Could you check a few things on this model? Use its own coordinates, in mm. A direction names the side the tool comes from. Coordinates: 2 decimals unless noted, no trailing zeros. Loops run counter-clockwise (first coordinate to the right, second up) from the corner with the lowest first, then second, coordinate; pieces in that order, holes last. Notation, with made-up numbers: (-20.5, -9.75) -> (-8.5, -9.75) arc R22 cw to (-8.5, 28.25) -> close; hole circle Ø1 at (-34.5, 89). An arc over 180 degrees is marked (long way). One line per question, with ' | ' between items.
from build123d import *

# Parameters (mm, degrees)
SKETCH3_W                   = 65
SKETCH3_H                   = 100
BOSS_EXTRUDE1_DEPTH         = 40
F_21_0_159_DIAMETER_HOLE1_D = 4.0386
SHELL1_T                    = -3.5
FILLET1_R                   = 2
SKETCH14_W                  = 13
SKETCH14_H                  = 7
CUT_EXTRUDE1_DEPTH          = 10
FILLET2_R                   = 5
CHAMFER2_SIZE               = 4
SKETCH15_R                  = 6.4
CUT_EXTRUDE3_DEPTH          = 10
SKETCH17_R                  = 6.4
CUT_EXTRUDE6_DEPTH          = 10
CUT_EXTRUDE8_DEPTH          = 1.5
SKETCH20_W                  = 51
SKETCH20_H                  = 53
BOSS_EXTRUDE3_DEPTH         = 17
SKETCH22_W                  = 49
SKETCH22_H                  = 49
CUT_EXTRUDE9_DEPTH          = 17
SKETCH23_R                  = 2.5
CUT_EXTRUDE10_DEPTH         = 3


with BuildPart() as part:
    # Sketch3 → Boss-Extrude1 (new body)
    with BuildSketch(Plane(origin=(0, 0, 0), x_dir=(1, 0, 0), z_dir=(0, 1, 0))):
        Rectangle(SKETCH3_W, SKETCH3_H)
    extrude(amount=BOSS_EXTRUDE1_DEPTH)

    # #21 (0.159) Diameter Hole1 (through all)
    with Locations(Plane(origin=(0, 40, 0), x_dir=(1, 0, 0), z_dir=(0, 1, 0))):
        with Locations((-26.15, 43.65), (26.15, 43.65), (26.15, -43.65), (-26.15, -43.65)):
            Hole(F_21_0_159_DIAMETER_HOLE1_D / 2)

    # Shell1
    shell1_openings = [part.faces().sort_by_distance(p)[0] for p in [
        (0, 40, 0),
    ]]
    offset(amount=SHELL1_T, openings=shell1_openings, kind=Kind.INTERSECTION)

    # Fillet1
    fillet1_edges = [part.edges().sort_by_distance(p)[0] for p in [
        (29, 21.75, 38.923460834),
        (21.423460834, 21.75, -46.5),
        (-29, 21.75, -38.923460834),
        (-21.423460834, 21.75, 46.5),
        (-29, 21.75, 38.923460834),
        (21.423460834, 21.75, 46.5),
        (29, 21.75, -38.923460834),
        (-21.423460834, 21.75, -46.5),
    ]]
    fillet(fillet1_edges, radius=FILLET1_R)

    # Sketch14 → Cut-Extrude1 (cut)
    with BuildSketch(Plane(origin=(0, 0, 0), x_dir=(1, 0, 0), z_dir=(0, 1, 0))):
        with Locations((-8.88380044, -40.5)):
            Rectangle(SKETCH14_W, SKETCH14_H)
        with Locations((9.11619956, -40.5)):
            Rectangle(SKETCH14_W, SKETCH14_H)
        with Locations((-8.88380044, 26.688454416)):
            Rectangle(SKETCH14_W, SKETCH14_H)
        with Locations((9.11619956, 26.688454416)):
            Rectangle(SKETCH14_W, SKETCH14_H)
    extrude(amount=CUT_EXTRUDE1_DEPTH, mode=Mode.SUBTRACT)

    # Fillet2
    fillet2_edges = [part.edges().sort_by_distance(p)[0] for p in [
        (32.5, 20, 50),
        (-32.5, 20, 50),
        (-32.5, 20, -50),
        (32.5, 20, -50),
    ]]
    fillet(fillet2_edges, radius=FILLET2_R)

    # Chamfer2
    chamfer2_edges = [part.edges().sort_by_distance(p)[0] for p in [
        (-31.035533906, 0, -48.535533906),
        (-31.035533906, 0, 48.535533906),
        (31.035533906, 0, -48.535533906),
        (31.035533906, 0, 48.535533906),
        (32.5, 0, 0),
    ]]
    chamfer(chamfer2_edges, length=CHAMFER2_SIZE)

    # Sketch15 → Cut-Extrude3 (cut)
    with BuildSketch(Plane(origin=(0, 0, -50), x_dir=(-1, 0, 0), z_dir=(0, 0, -1))):
        with Locations((0, 22)):
            Circle(SKETCH15_R)
    extrude(amount=-CUT_EXTRUDE3_DEPTH, mode=Mode.SUBTRACT)

    # Sketch17 → Cut-Extrude6 (cut)
    with BuildSketch(Plane(origin=(32.5, 0, 0), x_dir=(0, 0, -1), z_dir=(1, 0, 0))):
        with Locations((26.233387705, 29.113582019)):
            Circle(SKETCH17_R)
    extrude(amount=-CUT_EXTRUDE6_DEPTH, mode=Mode.SUBTRACT)

    # Sketch18 → Cut-Extrude8 (cut)
    with BuildSketch(Plane(origin=(0, 3.5, 0), x_dir=(1, 0, 0), z_dir=(0, 1, 0))):
        with BuildLine():
            Line((2.962903006, 35.660547198), (3, 35.660547198))
            Line((3, 35.660547198), (3, 31.660547198))
            Line((3, 31.660547198), (-3, 31.660547198))
            Line((-3, 31.660547198), (-3, 35.660547198))
            Line((-3, 35.660547198), (-2.962903006, 35.660547198))
            ThreePointArc((-2.962903006, 35.660547198), (0, 46.338397214), (2.962903006, 35.660547198))
        make_face()
    extrude(amount=-CUT_EXTRUDE8_DEPTH, mode=Mode.SUBTRACT)

    # Sketch20 → Boss-Extrude3 (add)
    with BuildSketch(Plane(origin=(0, 3.5, 0), x_dir=(1, 0, 0), z_dir=(0, 1, 0))):
        with Locations((3.5, -6.305895328)):
            Rectangle(SKETCH20_W, SKETCH20_H)
    extrude(amount=BOSS_EXTRUDE3_DEPTH)

    # Sketch22 → Cut-Extrude9 (cut)
    with BuildSketch(Plane(origin=(0, 20.5, 0), x_dir=(1, 0, 0), z_dir=(0, 1, 0))):
        with Locations((4.5, -6.305895328)):
            Rectangle(SKETCH22_W, SKETCH22_H)
    extrude(amount=-CUT_EXTRUDE9_DEPTH, mode=Mode.SUBTRACT)

    # Sketch23 → Cut-Extrude10 (cut)
    with BuildSketch(Plane.XY.offset(-18.194104672)):
        with Locations((-16.3, 8.5)):
            Circle(SKETCH23_R)
        with Locations((0, 8.5)):
            Circle(SKETCH23_R)
        with Locations((16.3, 8.5)):
            Circle(SKETCH23_R)
    extrude(amount=-CUT_EXTRUDE10_DEPTH, mode=Mode.SUBTRACT)


solid = part.part
1) I'm going to push flat-ended pins straight in: pin 1 Ø1.8 at (x, y) = (8.5, 1.5) entering from -Z; pin 2 Ø5 at (x, z) = (-18, 15) entering from +Y; pin 3 Ø1.6 at (y, z) = (2.5, -34) entering from +X. Where does each tip first touch, or does it pass through?
Data:
pin 1: z = -48.4 | pin 2: y = 20.5 | pin 3: x = 31.8
2) On a 3-axis mill with a long thin cutter (end or side, diameter ignored), from which of +Z, -Z, +X, -X, +Y, -Y can I reach the whole of each face in a straight line? I mean faces 4 (the face through (9, 2, 37)), 5 (the face through (-22, 12, 7)), 6 (the face through (-0.54, 6.06, -19.18)). Say none if no direction works.
Data:
face 4: +Y, -Y | face 5: +Y | face 6: none
3) If we section it at A-A on x = 10.5: Please give me the cut outline in (y, z).
Data:
outline: (0, -46) -> (4, -50) -> (40, -50) -> (40, -46.5) -> (3.5, -46.5) -> (3.5, -30.19) -> (0, -30.19) -> close; (0, -23.19) -> (3.5, -23.19) -> (3.5, -20.19) -> (20.5, -20.19) -> (20.5, -18.19) -> (3.5, -18.19) -> (3.5, 30.81) -> (20.5, 30.81) -> (20.5, 32.81) -> (3.5, 32.81) -> (3.5, 37) -> (0, 37) -> close; (0, 44) -> (3.5, 44) -> (3.5, 46.5) -> (40, 46.5) -> (40, 50) -> (4, 50) -> (0, 46) -> close
4) We'd pull the mould along Z, two halves only. Please class faces 1 (the face through (-29.62, 1.97, -47.08)), 2 (the face through (-29.58, 1.97, 47.12)), 3 (the face through (20, 21, -46)): pulls with the +Z half, pulls with the -Z half, needs draft (parallel to the pull), parting line crosses it, or undercut.
Data:
face 1: pulls with the -Z half | face 2: pulls with the +Z half | face 3: undercut
5) If we section it at C-C on y = 8.5: Give the number of separate pieces and of enclosed holes in the cut face, and give its area (3 significant figures).
Data:
separate pieces: 3 | enclosed holes: 5 | area: 1,570 mm²
6) I need wall thicknesses on line 1 along X through (y, z) = (15, 13); line 2 along Z through (x, y) = (-26.15, 26); line 3 along X through (y, z) = (27, -43.65). Which ranges of each line are inside material? Lowest first, please. Write a range as from..to.
Data:
line 1: -32.5..-29, -22..-20, 29..32.5 | line 2: -50..-45.67, -41.63..-38.13, 38.13..41.63, 45.67..50 | line 3: -32.5..-28.17, -24.13..-20.63, 20.63..24.13, 28.17..32.5
7) If we section it at B-B on z = -2: Please give me the cut outline in (x, y).
Data:
outline: (-32.5, 4) -> (-28.5, 0) -> (28.5, 0) -> (32.5, 4) -> (32.5, 40) -> (29, 40) -> (29, 3.5) -> (-20, 3.5) -> (-20, 20.5) -> (-22, 20.5) -> (-22, 3.5) -> (-29, 3.5) -> (-29, 40) -> (-32.5, 40) -> close
